```python
from build123d import *

# Parameters (mm, degrees)
SKETCH1_R           = 1.5
BOSS_EXTRUDE1_DEPTH = 3.175
CUT_EXTRUDE1_DEPTH  = 10


with BuildPart() as part:
    # Sketch1 → Boss-Extrude1 (new body)
    with BuildSketch(Plane(origin=(0, 0, 0), x_dir=(1, 0, 0), z_dir=(0, 1, 0))):
        with BuildLine():
            Line((7.858300919, -2.484134681), (13.014762042, -2.484134681))
            ThreePointArc((13.014762042, -2.484134681), (15.743606535, 0.244709812), (13.014762042, 2.973554305))
            Line((13.014762042, 2.973554305), (7.969118099, 2.744709812))
            ThreePointArc((7.969118099, 2.744709812), (5.624188125, 5.376129638), (2.206241257, 6.236772472))
            Line((2.206241257, 6.236772472), (-0.371989304, 10.702398798))
            ThreePointArc((-0.371989304, 10.702398798), (-4.099660205, 11.701225206), (-5.098486612, 7.973554305))
            Line((-5.098486612, 7.973554305), (-2.377479496, 3.718320719))
            ThreePointArc((-2.377479496, 3.718320719), (-3.483890927, 0.371841879), (-2.520256051, -3.018508355))
            Line((-2.520256051, -3.018508355), (-5.098486612, -7.484134681))
            ThreePointArc((-5.098486612, -7.484134681), (-4.099660205, -11.211805582), (-0.371989304, -10.212979174))
            Line((-0.371989304, -10.212979174), (1.952647522, -5.728901095))
            ThreePointArc((1.952647522, -5.728901095), (5.403988927, -5.013842081), (7.858300919, -2.484134681))
        make_face()
        Polygon((3.965354593, 2.757209812), (5.415947144, 0.244709812), (3.965354593, -2.267790188), (1.06416949, -2.267790188), (-0.386423061, 0.244709812), (1.06416949, 2.757209812), align=None, mode=Mode.SUBTRACT)
        with Locations(Location((13.014762042, 0.244709812, 0), (0, 0, 270))):
            Circle(SKETCH1_R, mode=Mode.SUBTRACT)
        with Locations(Location((-2.735237958, 9.337976552, 0), (0, 0, 270))):
            Circle(SKETCH1_R, mode=Mode.SUBTRACT)
        with Locations(Location((-2.735237958, -8.848556928, 0), (0, 0, 270))):
            Circle(SKETCH1_R, mode=Mode.SUBTRACT)
    extrude(amount=BOSS_EXTRUDE1_DEPTH)

    # Sketch2 → Cut-Extrude1 (cut)
    with BuildSketch(Plane(origin=(0, 3.175, 0), x_dir=(1, 0, 0), z_dir=(0, 1, 0))):
        Polygon((5.421720647, 0.244709812), (3.968241344, 2.762209812), (1.061282739, 2.762209812), (-0.392196564, 0.244709812), (1.061282739, -2.272790188), (3.968241344, -2.272790188), align=None)
    extrude(amount=-CUT_EXTRUDE1_DEPTH, mode=Mode.SUBTRACT)


solid = part.part
```
Model file for the job. Use its own axes, mm. A direction names the side the tool comes from. Coordinates: 2 decimals unless noted, no trailing zeros. Order: outer loops, then holes, each group sorted by start corner. A loop starts at its lowest first (then second) coordinate and runs counter-clockwise, first axis right, second up. Notation, with made-up numbers: (40.5, 62.25) -> (93.5, 62.25) arc R13 ccw to (93.5, 85.25) -> close; hole circle Ø10 at (-13.75, 4). An arc over 180 degrees is marked (long way). Answer as a JSON object with one key per item and string values. Group by question number.
1) Flat gauge pins, fed straight in: pin 1 (5 mm diameter, centred on x = -1, z = -4, fed in from -Y); pin 2 (1 mm diameter, centred on x = 0.5, y = 1.5, fed in from -Z); pin 3 (1 mm diameter, centred on x = 9, y = 1, fed in from +Z); pin 4 (0.9 mm diameter, centred on x = 2, y = 1.5, fed in from +Z). Where does each tip first touch, or does it go through?
2) Cut at C-C, the plane y = 2.4. Write the cut outline in (x, z).
3) Cut at A-A, the plane x = -3. Write the cut outline in (y, z) (3 decimals).
4) Which spindle directions (+Z, -Z, +X, -X, +Y, -Y) get a long thin tool onto all of the face, cutting with end or side? Do faces 4 (the face through (-3.76, 1.57, -5.88)), 5 (the face through (10, 2, 2.484)), 6 (the face through (4.705, 1.61, -1.486)). Say none if no direction does.
5) Drill centre lines: L1, parallel to Z at x = 13, y = 1.4; L2, parallel to Z at x = -1.5, y = 1.95; L3, parallel to X at y = 0.75, z = -1.25. Where is each one in solid material? Low to high.
6) Pull direction X, two halves, no side cores. Call faces 1 (the face through (3, 3.175, -3)), 2 (the face through (-4.05, 1.57, -11.73)), 3 (the face through (3, 2, -2.762)): +X half, -X half, draft (parallel to the pull), parting line (faces both ways), or undercut.
7) Cut at D-D, the plane x = 5. Write the cut outline in (y, z) (3 decimals).
8) Cut at B-B, the plane z = 9. Write the cut outline in (x, y) (3 decimals), then the cut area to 3 significant figures.
Check values:
{
 "1": {"pin 1": "stops at y = 0", "pin 2": "stops at z = -10.06", "pin 3": "stops at z = 2.48", "pin 4": "stops at z = 6.51"},
 "2": {"outline": "(-5.1, -7.97) arc R2.73 ccw to (-0.37, -10.7) -> (2.21, -6.24) arc R6 ccw to (7.97, -2.74) -> (13.01, -2.97) arc R2.73 ccw to (13.01, 2.48) -> (7.86, 2.48) arc R6 ccw to (1.95, 5.73) -> (-0.37, 10.21) arc R2.73 ccw to (-5.1, 7.48) -> (-2.52, 3.02) arc R6 ccw to (-2.38, -3.72) -> close; hole circle Ø3 at (-2.74, -9.34); hole circle Ø3 at (-2.74, 8.85); hole (-0.39, -0.24) -> (1.06, -2.76) -> (3.97, -2.76) -> (5.42, -0.24) -> (3.97, 2.27) -> (1.06, 2.27) -> close; hole circle Ø3 at (13.01, -0.24)"},
 "3": {"outline": "(0, -12.054) -> (3.175, -12.054) -> (3.175, -10.814) -> (0, -10.814) -> close; (0, -7.862) -> (3.175, -7.862) -> (3.175, -4.692) -> (0, -4.692) -> close; (0, -2.608) -> (3.175, -2.608) -> (3.175, 2.119) -> (0, 2.119) -> close; (0, 3.849) -> (3.175, 3.849) -> (3.175, 7.372) -> (0, 7.372) -> close; (0, 10.325) -> (3.175, 10.325) -> (3.175, 11.565) -> (0, 11.565) -> close"},
 "4": {"face 4": "-X, +Y, -Y", "face 5": "+Z, +X, +Y, -Y", "face 6": "+Y, -Y"},
 "5": {"L1": "z = -2.97 to -1.74, 1.26 to 2.48", "L2": "z = -11.77 to -10.19, -8.49 to 8, 9.7 to 11.28", "L3": "x = -3.4 to 0.19, 4.84 to 11.9, 14.13 to 15.55"},
 "6": {"face 1": "draft", "face 2": "parting line", "face 3": "undercut"},
 "7": {"outline": "(0, -5.706) -> (3.175, -5.706) -> (3.175, -0.975) -> (0, -0.975) -> close; (0, 0.486) -> (3.175, 0.486) -> (3.175, 5.216) -> (0, 5.216) -> close"},
 "8": {"outline": "(-5.46, 0) -> (-4.228, 0) -> (-4.228, 3.175) -> (-5.46, 3.175) -> close; (-1.243, 0) -> (0.257, 0) -> (0.257, 3.175) -> (-1.243, 3.175) -> close", "area": "8.67 mm²"}
}
